Geometry check sheet. Reference: the model listing, model coordinates, mm. A direction names the side the tool comes from. Give positions to 0.01 mm unless a question says otherwise; leave off trailing zeros. Write each loop counter-clockwise with the first axis right and the second up, starting at its lowest first coordinate (ties: lowest second). Pieces come first, ordered by that corner, then holes. Notation, with made-up numbers: (72.5, 62) - (109.5, 62) arc R32 ccw to (109.5, 97) - close; hole circle Ø2 at (34, 75.25). An arc over 180 degrees is marked (long way). One line per question, with ' | ' between items. Start each with the question number.
Q1. Thickness scan on L1, parallel to Y at x = 1, z = 1.2; L2, parallel to X at y = -29, z = 0.75; L3, parallel to Y at x = 30, z = 1.25. Record the ranges inside material, lowest first. Write a range as [from, to].
Q2. Set-up check for faces 1 (the face through (-38, 2, 1)), 2 (the face through (40, -16, 1)), 3 (the face through (7.5, 1, 2)), 4 (the face through (17.5, 41, 1)): record each of +Z, -Z, +X, -X, +Y, -Y from which the full face is reachable in a straight line by a thin tool's end or side.
Q3. Section check C-C on x = -32. Record the boundary of the cut face in (y, z), and give its area (3 significant figures).
Q4. Section check B-B on y = 29. Record the boundary of the cut face in (x, z).
Q5. Section check A-A on z = 1.45. Record the boundary of the cut face in (x, y), and give its area (3 significant figures).
Q6. Gauge pin test, flat ends, axial feed: P1, Ø1.5, axis at y = -33, z = 1.5, coming from the +X side; P2, Ø0.9, axis at x = 30, z = 1, coming from the +Y side; P3, Ø0.9, axis at y = 41.5, z = 2, coming from the +X side. Record the tip position at first contact, or that the pin passes through.
```python
from build123d import *

# Parameters (mm, degrees)
BOSS_EXTRUDE1_DEPTH = 3
SKETCH2_W           = 15
SKETCH2_H           = 3
CUT_EXTRUDE1_DEPTH  = 3


with BuildPart() as part:
    # Sketch1 → Boss-Extrude1 (new body)
    with BuildSketch(Plane.XY):
        Polygon((-38, 39.5), (-17.5, 39.5), (-17.5, 42.5), (17.5, 42.5), (17.5, 39.5), (38, 39.5), (38, 19), (41, 19), (41, 16), (41, -16), (38, -16), (38, -19), (38, -39.5), (-41, -39.5), (-41, -19), (-41, -16), (-38, -16), (-38, 16), (-38, 19), (-41, 19), (-41, 39.5), align=None)
    extrude(amount=BOSS_EXTRUDE1_DEPTH)

    # Sketch2 → Cut-Extrude1 (cut)
    with BuildSketch(Plane.XY.offset(3)):
        with Locations((0, 1.5)):
            Rectangle(SKETCH2_W, SKETCH2_H)
    extrude(amount=-CUT_EXTRUDE1_DEPTH, mode=Mode.SUBTRACT)


solid = part.part
```
Working result:
1) L1: y = [-39.5, 0], [3, 42.5] | L2: x = [-41, 38] | L3: y = [-39.5, 39.5]
2) face 1: +Z, -Z, -X | face 2: +Z, -Z, +X, -Y | face 3: +Z, -Z | face 4: +Z, -Z, +X, +Y
3) outline: (-39.5, 0) - (39.5, 0) - (39.5, 3) - (-39.5, 3) - close | area: 237 mm2
4) outline: (-41, 0) - (38, 0) - (38, 3) - (-41, 3) - close
5) outline: (-41, -39.5) - (38, -39.5) - (38, -16) - (41, -16) - (41, 19) - (38, 19) - (38, 39.5) - (17.5, 39.5) - (17.5, 42.5) - (-17.5, 42.5) - (-17.5, 39.5) - (-41, 39.5) - (-41, 19) - (-38, 19) - (-38, -16) - (-41, -16) - close; hole (-7.5, 0) - (7.5, 0) - (7.5, 3) - (-7.5, 3) - close | area: 6,300 mm2
6) P1: stops at x = 38 | P2: stops at y = 39.5 | P3: stops at x = 17.5
